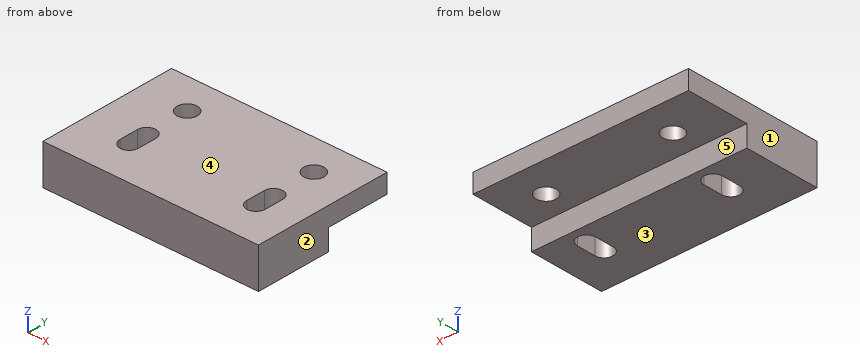
Autodesk Inventor part; units mm, degrees
ref_plane "Work Plane2" through (-108.8568, -31.2741, 3.325) normal (0, 0, 1) x (0.8192, 0.5736, 0)
ref_plane "YZ Plane" through (0, 0, 0) normal (1, 0, 0) x (0, 1, 0)
ref_plane "XZ Plane" through (0, 0, 0) normal (0, 1, 0) x (-1, 0, 0)
ref_plane "Work Plane1" through (0, 0, 0) normal (0, 0, 1) x (1, 0, 0)
sketch "Sketch1" plane through (0, 0, 0) normal (0, 0, 1) x (1, 0, 0)
  circle A0 centre (-24.675, -5.1) radius 1.25
  circle A1 centre (-4.675, -5.1) radius 1.25
  line L0 (-32.4114, -2.1) -> (22.9321, -2.1) construction
  line L1 (-32.4114, -2.4674) -> (1.5886, -2.4674)
  line L2 (1.5886, -2.4674) -> (1.5886, -14.4674)
  line L3 (1.5886, -14.4674) -> (-32.4114, -14.4674)
  line L4 (-32.4114, -14.4674) -> (-32.4114, -2.4674)
  circle A2 centre (-24.675, -5.1) radius 1.45
  circle A3 centre (-4.675, -5.1) radius 1.45
  line L5 (-24.675, -5.1) -> (-24.675, -8.1)
  line L6 (-23.225, -5.1) -> (-23.225, -8.1)
  line L7 (-26.125, -8.1) -> (-26.125, -5.1)
  arc A4 (-23.225, -5.1) -> (-26.125, -5.1) centre (-24.675, -5.1) ccw
  arc A5 (-26.125, -8.1) -> (-23.225, -8.1) centre (-24.675, -8.1) ccw
  line L8 (-4.675, -5.1) -> (-4.675, -8.1)
  line L9 (-6.125, -5.1) -> (-6.125, -8.1)
  line L10 (-3.225, -8.1) -> (-3.225, -5.1)
  arc A6 (-3.225, -5.1) -> (-6.125, -5.1) centre (-4.675, -5.1) ccw
  arc A7 (-6.125, -8.1) -> (-3.225, -8.1) centre (-4.675, -8.1) ccw
  point P0 (0, 0)
  point P1 (-24.675, -6.6)
  point P2 (-4.675, -6.6)
  dimension "d0" = 34
  dimension "d1" = 12
  dimension "d2" = 2.9
  dimension "d3" = 2.9
  dimension "d4" = 3
  dimension "d5" = 3
ref_plane "Work Plane2" through (-108.8568, -31.2741, 3.325) normal (0, 0, 1) x (0.8192, 0.5736, 0)
extrude "Extrusion1" add sketch "Sketch1" along normal up to surface (3.325 mm away) contours L1 L2 L3 L4
sketch "Sketch2" plane through (-32.4114, -2.4674, 3.325) normal (0, 0, 1) x (1, 0, 0)
  circle A0 centre (27.7364, 4.2761) radius 1.6
  circle A1 centre (7.7364, 4.2761) radius 1.6
  line L0 (-8.2471, 157.2957) -> (-14.2937, 153.0618)
  line L1 (8.339, 104.3183) -> (-14.2937, 153.0618)
  line L2 (8.339, 104.3183) -> (0.8847, 99.0987)
  line L3 (0.8847, 99.0987) -> (0, 100.3623)
  line L4 (0, 100.3623) -> (0, 0.3674)
  line L5 (0, 0.3674) -> (55.3435, 0.3674)
  line L6 (55.3435, 0.3674) -> (57.5639, -2.8038)
  line L7 (57.5639, -2.8038) -> (65.7554, 2.932)
  line L8 (65.7554, 2.932) -> (31.3409, 52.0811)
  line L9 (31.3409, 52.0811) -> (41.1707, 58.964)
  line L10 (41.1707, 58.964) -> (36.2423, 66.0024)
  arc A2 (34.9764, 70.0175) -> (36.2423, 66.0024) centre (41.9764, 70.0175) ccw
  line L11 (34.9764, 70.0175) -> (34.9764, 131.4195)
  arc A3 (34.9764, 131.4195) -> (31.2086, 137.6285) centre (27.9764, 131.4195) ccw
  line L12 (31.2086, 137.6285) -> (10.9451, 148.1771)
  arc A4 (10.9451, 148.1771) -> (3.6978, 147.7021) centre (7.7129, 141.968) ccw
  line L13 (3.6978, 147.7021) -> (0.1902, 145.246)
  line L14 (-8.2471, 157.2957) -> (0.1902, 145.246)
  line L15 (6.7364, -8.3116) -> (6.7364, -9.6116)
  line L16 (7.7364, -12.1836) -> (7.7364, -9.6116)
  line L17 (34, 0) -> (34, -12)
  line L18 (0, 0) -> (34, 0)
  line L19 (0, -12) -> (0, 0)
  line L20 (34, -12) -> (0, -12)
  arc A5 (6.2864, -5.6326) -> (9.1864, -5.6326) centre (7.7364, -5.6326) ccw
  line L21 (6.2864, -2.6326) -> (6.2864, -5.6326)
  arc A6 (9.1864, -2.6326) -> (6.2864, -2.6326) centre (7.7364, -2.6326) ccw
  line L22 (9.1864, -5.6326) -> (9.1864, -2.6326)
  arc A7 (29.1864, -2.6326) -> (26.2864, -2.6326) centre (27.7364, -2.6326) ccw
  line L23 (29.1864, -5.6326) -> (29.1864, -2.6326)
  arc A8 (26.2864, -5.6326) -> (29.1864, -5.6326) centre (27.7364, -5.6326) ccw
  line L24 (26.2864, -2.6326) -> (26.2864, -5.6326)
  line L25 (0, 0) -> (34, 0)
  line L26 (0, 0) -> (34, 0)
  line L27 (34, 0) -> (34, 10)
  line L28 (34, 10) -> (0, 10)
  line L29 (0, 10) -> (0, 0)
  point P0 (32.4114, 2.4674)
  dimension "d8" = 10
extrude "Extrusion2" add sketch "Sketch2" along normal blind 3 contours L28 L27 L5 L4 | L5 L27 L18 L29 | L18 L17 L20 L19
properties part number "cellSTORM_Alvium_cameraadapter"
Verification items for the finished model (mm, model axes). Face numbers are marked on the shaded views. A direction names the side the tool comes from. Round coordinates to 2 decimals unless told otherwise and drop trailing zeros. Write each loop counter-clockwise with the first axis right and the second up, starting at its lowest first coordinate (ties: lowest second). Pieces come first, ordered by that corner, then holes. Notation, with made-up numbers: (34.25, -38.75) -> (84.25, -38.75) arc R27 cw to (84.25, -10.75) -> close; hole circle Ø8 at (-25, -6). An arc over 180 degrees is marked (long way). Write each question's results on one line, items separated by ' | '. Start each with the question number.
1. Cross-section at B-B (z = 2). Enter the section's corners in (x, y) (3 decimals), then the cut area to 3 significant figures.
2. Draft check along X on the marked faces 1, 2 and 3. Enter one of: +X half, -X half, draft (parallel to the pull), parting line (faces both ways), or undercut.
3. Cross-section at A-A (y = -6.25). Enter the section's corners in (x, z) (3 decimals).
4. Cross-section at D-D (x = -28). Enter the section's corners in (y, z) (3 decimals).
5. Depth check by flat-ended pin: P1, Ø5, axis at x = -29, y = 3.5, coming from the -Z side (3 decimals); P2, Ø1, axis at x = -14.5, z = 2, coming from the +Y side. Enter the tip coordinate at first touch or a pass-through.
6. Set-up check for the marked faces 4 and 5: record each of +Z, -Z, +X, -X, +Y, -Y from which the full face is reachable in a straight line by a thin tool's end or side.
7. Material ranges on probe 1 along X at (y, z) = (-7, 3.75) (3 decimals); probe 2 along X at (y, z) = (-8.5, 1.5); probe 3 along Y at (x, z) = (-2, 2), recorded low to high. Write a range as from..to.
8. Cross-section at C-C (x = -5.5). Enter the section's corners in (y, z) (3 decimals), then the cut area to 3 significant figures.
Solutions:
1) outline: (-32.411, -14.467) -> (1.589, -14.467) -> (1.589, -2.467) -> (-32.411, -2.467) -> close; hole (-26.125, -8.1) arc R1.45 ccw to (-23.225, -8.1) -> (-23.225, -5.1) arc R1.45 ccw to (-26.125, -5.1) -> close; hole (-6.125, -8.1) arc R1.45 ccw to (-3.225, -8.1) -> (-3.225, -5.1) arc R1.45 ccw to (-6.125, -5.1) -> close | area: 377 mm2
2) face 1: -X half | face 2: +X half | face 3: draft
3) outline: (-32.411, 0) -> (-26.125, 0) -> (-26.125, 6.325) -> (-32.411, 6.325) -> close; (-23.225, 0) -> (-6.125, 0) -> (-6.125, 6.325) -> (-23.225, 6.325) -> close; (-3.225, 0) -> (1.589, 0) -> (1.589, 6.325) -> (-3.225, 6.325) -> close
4) outline: (-14.467, 0) -> (-2.467, 0) -> (-2.467, 3.325) -> (7.533, 3.325) -> (7.533, 6.325) -> (-14.467, 6.325) -> close
5) P1: stops at z = 3.325 | P2: stops at y = -2.47
6) face 4: +Z, +X, -X, +Y, -Y | face 5: -Z, +X, -X, +Y
7) probe 1: x = -32.411..-26.125, -23.225..-6.125, -3.225..1.589 | probe 2: x = -32.41..-26.07, -23.28..-6.07, -3.28..1.59 | probe 3: y = -14.47..-2.47
8) outline: (-14.467, 0) -> (-9.292, 0) -> (-9.292, 6.325) -> (-14.467, 6.325) -> close; (-3.908, 0) -> (-2.467, 0) -> (-2.467, 3.325) -> (0.438, 3.325) -> (0.438, 6.325) -> (-3.908, 6.325) -> close; (3.18, 3.325) -> (7.533, 3.325) -> (7.533, 6.325) -> (3.18, 6.325) -> close | area: 63.6 mm2
